Geometry: final body of the model. Coordinates: model frame, mm. Give positions to 0.01 mm unless a question says otherwise; leave off trailing zeros. Write each loop counter-clockwise with the first axis right and the second up, starting at its lowest first coordinate (ties: lowest second). Pieces come first, ordered by that corner, then holes. Notation, with made-up numbers: (43.25, -17.5) -> (50.25, -17.5) arc R19 cw to (50.25, -6.5) -> close; hole circle Ø7 at (39.25, -31). An arc over 180 degrees is marked (long way). Answer as a JSON object with one key per item and string values.
from build123d import *

# Parameters (mm, degrees)
BOSS_EXTRUDE1_DEPTH = 2.5
SKETCH3_R           = 3
BOSS_EXTRUDE2_DEPTH = 14
SKETCH4_R           = 3.25
BOSS_EXTRUDE3_DEPTH = 9


with BuildPart() as part:
    # Sketch2 → Boss-Extrude1 (new body)
    with BuildSketch(Plane.XY):
        with BuildLine():
            Line((-50.233491964, 44.055695146), (79.766508036, 44.055695146))
            ThreePointArc((79.766508036, 44.055695146), (86.837575848, 41.126762958), (89.766508036, 34.055695146))
            Line((89.766508036, 34.055695146), (89.766508036, -95.944304854))
            ThreePointArc((89.766508036, -95.944304854), (86.837575848, -103.015372665), (79.766508036, -105.944304854))
            Line((79.766508036, -105.944304854), (-50.233491964, -105.944304854))
            ThreePointArc((-50.233491964, -105.944304854), (-57.304559776, -103.015372665), (-60.233491964, -95.944304854))
            Line((-60.233491964, -95.944304854), (-60.233491964, 34.055695146))
            ThreePointArc((-60.233491964, 34.055695146), (-57.304559776, 41.126762958), (-50.233491964, 44.055695146))
        make_face()
    extrude(amount=BOSS_EXTRUDE1_DEPTH)

    # Sketch3 → Boss-Extrude2 (add)
    with BuildSketch(Plane.XY.offset(2.5)):
        with Locations(Location((-52.733491964, 35.055695146, 0), (0, 0, 180))):
            Circle(SKETCH3_R)
        with Locations(Location((-52.733491964, -15.944304854, 0), (0, 0, 180))):
            Circle(SKETCH3_R)
        with Locations(Location((82.266508036, -15.944304854, 0), (0, 0, 180))):
            Circle(SKETCH3_R)
        with Locations(Location((82.266508036, 35.055695146, 0), (0, 0, 180))):
            Circle(SKETCH3_R)
    extrude(amount=BOSS_EXTRUDE2_DEPTH)

    # Sketch4 → Boss-Extrude3 (add)
    with BuildSketch(Plane.XY.offset(2.5)):
        with Locations(Location((80.766508036, -98.444304854, 0), (0, 0, 180))):
            Circle(SKETCH4_R)
    extrude(amount=BOSS_EXTRUDE3_DEPTH)


solid = part.part
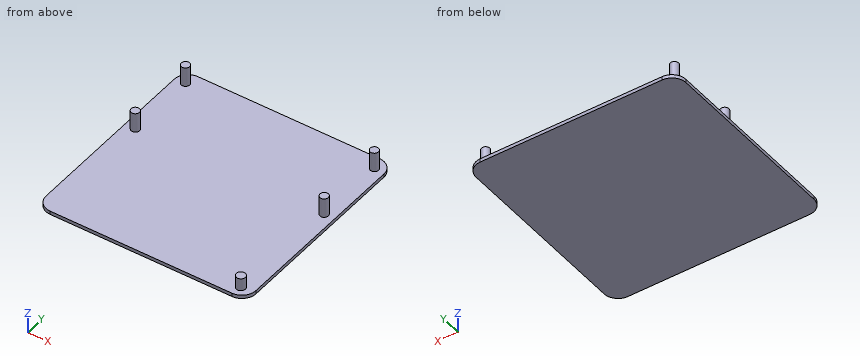
Q1. Material intervals for L1, parallel to Z at x = 54.5, y = -73, sorted ascending. Write a range as from..to.
Values:
{"L1": "0..2.5"}
Q2. Cut plane B-B (z = 14.5). Return the cut outline in (x, y).
Values:
{"outline": "circle Ø6 at (-52.73, -15.94); circle Ø6 at (-52.73, 35.06); circle Ø6 at (82.27, -15.94); circle Ø6 at (82.27, 35.06)"}
Q3. First-contact query: P1, Ø5, axis at x = 82, y = -97.5, coming from the +Z side; P2, Ø2, axis at y = 27.5, z = 5, coming from the +X side; P3, Ø10, axis at x = 53, y = 28, coming from the +Z side. Flat tips, straight axial feed; report the tip coordinate or a pass-through.
Values:
{"P1": "z = 11.5", "P2": "through", "P3": "z = 2.5"}
Q4. Cut plane C-C (y = 28.5). Return the cut outline in (x, z), and give its area (3 significant figures).
Values:
{"outline": "(-60.23, 0) -> (89.77, 0) -> (89.77, 2.5) -> (-60.23, 2.5) -> close", "area": "375 mm²"}
Q5. Cut plane A-A (x = 18). Return the cut outline in (y, z).
Values:
{"outline": "(-105.94, 0) -> (44.06, 0) -> (44.06, 2.5) -> (-105.94, 2.5) -> close"}
